Part model, mm, in its own coordinate system. Face numbers are marked on the shaded views. A direction names the side the tool comes from. Coordinates: 2 decimals unless noted, no trailing zeros. Loops run counter-clockwise (first coordinate to the right, second up) from the corner with the lowest first, then second, coordinate; pieces in that order, holes last. Notation, with made-up numbers: (6.5, -29) - (18.5, -29) arc R5 ccw to (18.5, -22) - close; hole circle Ø9 at (55, 40.25). An arc over 180 degrees is marked (long way). Answer as CSV lines item,"result".
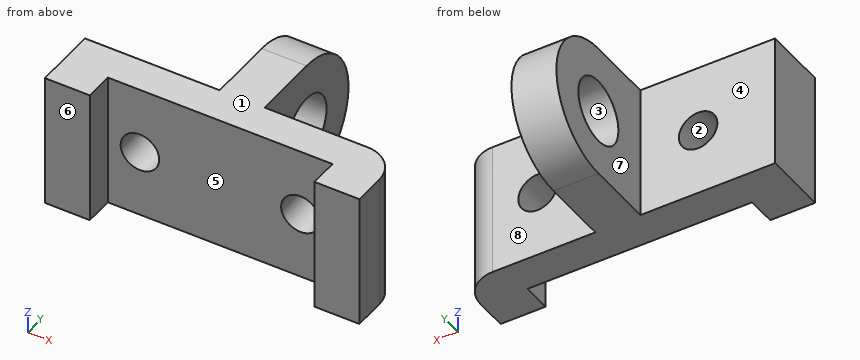
from build123d import *

# Parameters (mm, degrees)
SKETCH1_W           = 98
SKETCH1_H           = 42
BOSS_EXTRUDE1_DEPTH = 20
SKETCH2_W           = 70
SKETCH2_H           = 9
CUT_EXTRUDE1_DEPTH  = 68.564783726
SKETCH3_W           = 14
SKETCH3_H           = 42
BOSS_EXTRUDE2_DEPTH = 21
SKETCH4_R           = 21
BOSS_EXTRUDE3_DEPTH = 14
SKETCH5_R           = 6
CUT_EXTRUDE2_DEPTH  = 68.867518004
FILLET3_R           = 10
SKETCH6_R           = 10
CUT_EXTRUDE3_DEPTH  = 14


with BuildPart() as part:
    # Sketch1 → Boss-Extrude1 (new body)
    with BuildSketch(Plane(origin=(0, 0, 0), x_dir=(1, 0, 0), z_dir=(0, 1, 0))):
        Rectangle(SKETCH1_W, SKETCH1_H)
    extrude(amount=BOSS_EXTRUDE1_DEPTH)

    # Sketch2 → Cut-Extrude1 (cut, through all)
    with BuildSketch(Plane.XY.offset(21)):
        with Locations((0, 4.5)):
            Rectangle(SKETCH2_W, SKETCH2_H)
    extrude(amount=-CUT_EXTRUDE1_DEPTH, mode=Mode.SUBTRACT)

    # Sketch3 → Boss-Extrude2 (add)
    with BuildSketch(Plane(origin=(0, 20, 0), x_dir=(1, 0, 0), z_dir=(0, 1, 0))):
        Rectangle(SKETCH3_W, SKETCH3_H)
    extrude(amount=BOSS_EXTRUDE2_DEPTH)

    # Sketch4 → Boss-Extrude3 (add)
    with BuildSketch(Plane(origin=(7, 0, 0), x_dir=(0, 0, -1), z_dir=(1, 0, 0))):
        with Locations((0, 41)):
            Circle(SKETCH4_R)
    extrude(amount=-BOSS_EXTRUDE3_DEPTH)

    # Sketch5 → Cut-Extrude2 (cut, through all)
    with BuildSketch(Plane(origin=(0, 20, 0), x_dir=(1, 0, 0), z_dir=(0, 1, 0))):
        with Locations(Location((25, 0, 0), (0, 0, 270))):
            Circle(SKETCH5_R)
    cut_extrude2 = extrude(amount=-CUT_EXTRUDE2_DEPTH, mode=Mode.SUBTRACT)

    # Mirror1: Cut-Extrude2 across plane
    add(cut_extrude2.mirror(Plane(origin=(0, 0, 0), x_dir=(0, 0, 1), z_dir=(1, 0, 0))), mode=Mode.SUBTRACT)

    # Fillet3
    fillet3_edges = [part.edges().sort_by_distance(p)[0] for p in [
        (49, 20, 0),
    ]]
    fillet(fillet3_edges, radius=FILLET3_R)

    # Sketch6 → Cut-Extrude3 (cut)
    with BuildSketch(Plane(origin=(7, 0, 0), x_dir=(0, 0, -1), z_dir=(1, 0, 0))):
        with Locations((0, 41)):
            Circle(SKETCH6_R)
    extrude(amount=-CUT_EXTRUDE3_DEPTH, mode=Mode.SUBTRACT)


solid = part.part
Q1. Saw through at D-D (y = 18.5). Give the cut face in (x, z), then the cut area to 3 significant figures.
Results:
outline,"(-49, -21) - (44.27, -21) - (44.27, 21) - (-49, 21) - close; hole circle Ø12 at (-25, 0); hole circle Ø12 at (25, 0)"
area,"3,690 mm^2"
Q2. Flat gauge pins, fed straight in: pin 1 (10 mm diameter, centred on y = 40, z = 5.5, fed in from +X); pin 2 (1.5 mm diameter, centred on x = 16, z = 12.5, fed in from +Y); pin 3 (4 mm diameter, centred on y = 49.5, z = -15.5, fed in from -X). Where does each tip first touch, or does it go through?
Results:
pin 1,"stops at x = 7"
pin 2,"stops at y = 20"
pin 3,"stops at x = -7"
Q3. Saw through at B-B (y = 33.5). Give the cut face in (x, z).
Results:
outline,"(-7, -21) - (7, -21) - (7, -6.61) - (-7, -6.61) - close; (-7, 6.61) - (7, 6.61) - (7, 21) - (-7, 21) - close"
Q4. Saw through at C-C (x = -25). Give the cut face in (y, z), then the cut area to 3 significant figures.
Results:
outline,"(9, -21) - (20, -21) - (20, -6) - (9, -6) - close; (9, 6) - (20, 6) - (20, 21) - (9, 21) - close"
area,"330 mm^2"
Q5. Which spindle directions (+Z, -Z, +X, -X, +Y, -Y) get a long thin tool onto all of the face, cutting with end or side? Do the marked faces 5, 6, 7 and 8. Say none if no direction does.
Results:
face 5,"+Z, -Z, -Y"
face 6,"+Z, -Z, +X, -X, -Y"
face 7,"+Z, -Z, -X, +Y"
face 8,"+Z, -Z, +X, +Y"
Q6. Saw through at A-A (z = 0). Give the cut face in (x, y).
Results:
outline,"(-49, 0) - (-35, 0) - (-35, 9) - (-31, 9) - (-31, 20) - (-49, 20) - close; (-19, 9) - (19, 9) - (19, 20) - (7, 20) - (7, 31) - (-7, 31) - (-7, 20) - (-19, 20) - close; (-7, 51) - (7, 51) - (7, 62) - (-7, 62) - close; (31, 9) - (35, 9) - (35, 0) - (49, 0) - (49, 10) arc R10 ccw to (39, 20) - (31, 20) - close"
Q7. Wall check: L1, parallel to Z at x = 0, y = 33; L2, parallel to X at y = 12.5, z = 0; L3, parallel to Y at x = 0.5, z = 0. Give the ranges that are in metal, low to high.
Results:
L1,"z = -21 to -6, 6 to 21"
L2,"x = -49 to -31, -19 to 19, 31 to 48.68"
L3,"y = 9 to 31, 51 to 62"
Q8. Two-plate mould, pull along Z, no slides. Class the marked faces 1, 2, 3 and 4: released by +Z, released by -Z, zero draft, split by the parting line, or undercut.
Results:
face 1,"released by +Z"
face 2,"undercut"
face 3,"undercut"
face 4,"zero draft"
